```python
from build123d import *

# Parameters (mm, degrees)
F0_W     = 25.4
F0_H     = 25.4
F1_DEPTH = 38.1
F2_R     = 3.1962081395
F3_DEPTH = 12.7
F4_SIZE  = 12.69999
F5_R     = 2.54


# Not quite as in the source:
# - a fillet or chamfer is up to 0.001 mm smaller than in the source, because OpenCascade refuses the exact size


with BuildPart() as f1:
    # F0 (on Front) → F1 (new body)
    with BuildSketch(Plane.XZ):
        with Locations((-10.8844147762, 4.0432729903)):
            Rectangle(F0_W, F0_H)
    extrude(amount=F1_DEPTH)

    # F2 (on face) → F3 (join)
    with BuildSketch(Plane.XZ.offset(38.1)):
        with Locations((-10.8844147762, 4.0432729903)):
            Circle(F2_R)
    extrude(amount=F3_DEPTH)

    # F4 (size 12.7 in the source; OpenCascade refuses exactly that, so slightly less here)
    f4_edges = [f1.edges().sort_by_distance(p)[0] for p in [
        (-10.884415, 0, 16.743273),
        (-10.884415, 0, -8.656727),
        (1.815585, 0, 4.043273),
        (-23.584415, 0, 4.043273),
    ]]
    chamfer(f4_edges, length=F4_SIZE)

    # F5
    f5_edges = [f1.edges().sort_by_distance(p)[0] for p in [
        (-23.584415, -12.69999, 4.043273),
        (-10.884415, -12.69999, 16.743273),
        (1.815585, -12.69999, 4.043273),
        (-10.884415, -12.69999, -8.656727),
    ]]
    fillet(f5_edges, radius=F5_R)


solid = f1.part
```
CAD build for the part. Positions are in the model's coordinates, mm. A direction names the side the tool comes from. Coordinates: 2 decimals unless noted, no trailing zeros. Order: outer loops, then holes, each group sorted by start corner. A loop starts at its lowest first (then second) coordinate and runs counter-clockwise, first axis right, second up.
(1) Saw through at C-C, the plane y = -42.5. Write the cut outline in (x, z).
Solution:
outline: circle Ø6.39 at (-10.88, 4.04)
(2) Saw through at D-D, the plane x = -12.5. Write the cut outline in (y, z), and give its area (3 significant figures).
Solution:
outline: (-50.8, 1.29) - (-38.1, 1.29) - (-38.1, -8.66) - (-13.75, -8.66) arc R2.54 ccw to (-11.96, -7.91) - (-1.62, 2.43) - (-1.62, 5.66) - (-11.96, 16) arc R2.54 ccw to (-13.75, 16.74) - (-38.1, 16.74) - (-38.1, 6.8) - (-50.8, 6.8) - close
area: 874 mm2
(3) Saw through at B-B, the plane x = -19. Write the cut outline in (y, z), and give its area (3 significant figures).
Solution:
outline: (-38.1, -8.66) - (-13.75, -8.66) arc R2.54 ccw to (-11.96, -7.91) - (-8.12, -4.07) - (-8.12, 12.16) - (-11.96, 16) arc R2.54 ccw to (-13.75, 16.74) - (-38.1, 16.74) - close
area: 740 mm2
(4) Which spindle directions (+Z, -Z, +X, -X, +Y, -Y) get a long thin tool onto all of the face, cutting with end or side? Do faces 1 (the face through (-18.107, -7.223, 3.876)), 2 (the face through (-7.836, -44.361, 5.003)). Say none if no direction does.
Solution:
face 1: +Z, -Z, -X, +Y
face 2: -Y
(5) Drill centre lines: L1, parallel to Y at x = -0.75, z = 2.75; L2, parallel to Y at x = -6.5, z = 15; L3, parallel to X at y = -41.5, z = 1.25. Where is each one in solid material? Low to high.
Solution:
L1: y = -38.1 to -10.13
L2: y = -38.1 to -10.96
L3: x = -12.44 to -9.33
(6) Saw through at A-A, the plane z = -1. Write the cut outline in (x, y).
Solution:
outline: (-23.58, -38.1) - (1.82, -38.1) - (1.82, -13.75) arc R2.54 ccw to (1.07, -11.96) - (-5.84, -5.04) - (-15.93, -5.04) - (-22.84, -11.96) arc R2.54 ccw to (-23.58, -13.75) - close
(7) Pin check, flat tips, straight feed: pin 1 Ø6 at (y, z) = (-42.5, 11) entering from +X; pin 2 Ø12 at (x, y) = (-8.5, -45) entering from -Z; pin 3 Ø6 at (x, z) = (-19.5, 3.5) entering from +Y; pin 4 Ø3 at (x, z) = (-12, 12.5) entering from -Y. Stop position of each tip, or through.
Solution:
pin 1: passes through
pin 2: stops at z = 0.85
pin 3: stops at y = -5.62
pin 4: stops at y = -38.1
